The listing builds one solid part. Answer for the finished solid, in the listing's coordinates (mm). Give positions to 0.01 mm unless a question says otherwise; leave off trailing zeros. Order: outer loops, then holes, each group sorted by start corner. A loop starts at its lowest first (then second) coordinate and runs counter-clockwise, first axis right, second up. Notation, with made-up numbers: (57.25, -10) - (102.25, -10) arc R5 cw to (102.25, -4) - close; hole circle Ø6 at (-10, 15.5). An arc over 180 degrees is marked (long way). Answer as a JSON object with one key per item and string values. Group by question number.
Q1. A cutting plane is placed at C-C, the plane z = 5.05. Give the vertices of the cut face in (x, y).
Q2. Consider line 1 (Y direction, x = 9.5, z = 4.15); line 2 (X direction, y = 8.5, z = 1.9); line 3 (Y direction, x = -9.5, z = 0.6). Determine where each line is inside the solid, lowest interval first.
Q3. A cutting plane is placed at A-A, the plane x = -12. Give the vertices of the cut face in (y, z), and give its area (3 significant figures).
from build123d import *

# Parameters (mm, degrees)
SKETCH_W  = 30
SKETCH_H  = 30
PAD_DEPTH = 6
FILLET_R  = 2


with BuildPart() as part:
    # Sketch → Pad (new body)
    with BuildSketch(Plane.XY):
        Rectangle(SKETCH_W, SKETCH_H)
    extrude(amount=PAD_DEPTH)

    # Fillet
    fillet_edges = [part.edges().sort_by_distance(p)[0] for p in [
        (0, -15, 6),
        (-15, 0, 6),
        (0, 15, 6),
        (15, 0, 6),
        (-15, 0, 0),
        (0, -15, 0),
        (0, 15, 0),
        (15, 0, 0),
    ]]
    fillet(fillet_edges, radius=FILLET_R)


solid = part.part
Reply:
{
 "1": {"outline": "(-14.7, -14.7) - (14.7, -14.7) - (14.7, 14.7) - (-14.7, 14.7) - close"},
 "2": {"line 1": "y = -14.99 to 14.99", "line 2": "x = -15 to 15", "line 3": "y = -14.43 to 14.43"},
 "3": {"outline": "(-15, 2) arc R2 ccw to (-13, 0) - (13, 0) arc R2 ccw to (15, 2) - (15, 4) arc R2 ccw to (13, 6) - (-13, 6) arc R2 ccw to (-15, 4) - close", "area": "177 mm^2"}
}
